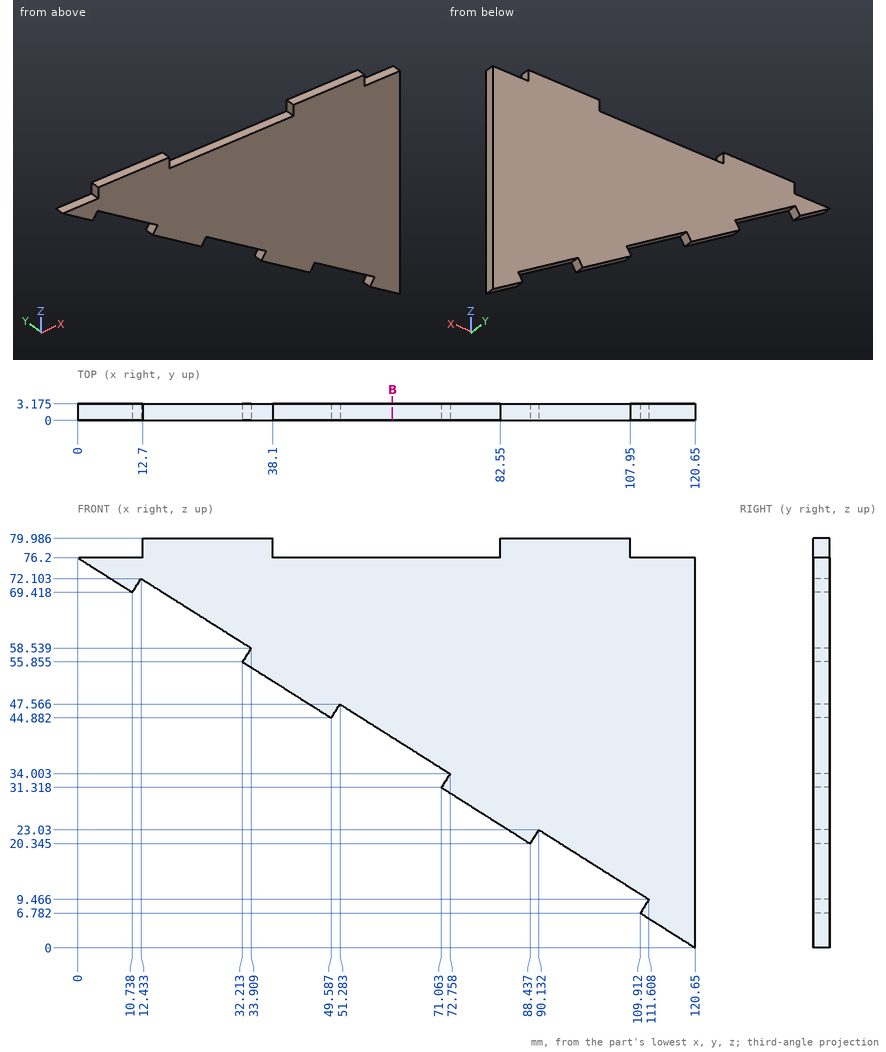
Part print with two shaded views. Sizes in mm from the minimum x, y, z corner. Give positions to 0.01 mm unless a question says otherwise; leave off trailing zeros. Write each loop counter-clockwise with the first axis right and the second up, starting at its lowest first coordinate (ties: lowest second). Pieces come first, ordered by that corner, then holes.
1) Cut at B-B on x = 61.5. Write the cut outline in (y, z) (1 decimal), then the cut area to 3 significant figures.
Resolved:
outline: (0, 41.1) - (3.2, 41.1) - (3.2, 76.2) - (0, 76.2) - close
area: 111 mm2
2) Probe L1, parallel to Z at x = 33, y = 2.55 (1 decimal); L2, parallel to Z at x = 73, y = 1 (1 decimal); L3, parallel to Z at x = 81.5, y = 2.1 (1 decimal). List the from-to ranges inside material, lowest first.
Resolved:
L1: z = 55.4 to 57.1, 59.1 to 80
L2: z = 30.1 to 76.2
L3: z = 24.7 to 76.2
3) Pin check, flat tips, straight feed: pin 1 (4 mm diameter, centred on x = 93, z = 70.5, fed in from -Y); pin 2 (1.6 mm diameter, centred on y = 1, z = 78.5, fed in from -X); pin 3 (1.6 mm diameter, centred on y = 1.5, z = 78.5, fed in from +X); pin 4 (1.6 mm diameter, centred on x = 115, y = 1, fed in from +Z). Stop position of each tip, or through.
Resolved:
pin 1: stops at y = 0
pin 2: stops at x = 12.7
pin 3: stops at x = 107.95
pin 4: stops at z = 76.2
